For this review, take the finished solid that the model builds, in its own axes (mm). A direction names the side the tool comes from. Coordinates: 2 decimals unless noted, no trailing zeros. Loops run counter-clockwise (first coordinate to the right, second up) from the corner with the lowest first, then second, coordinate; pieces in that order, holes last. Notation, with made-up numbers: (35, 32) - (57, 32) arc R24 ccw to (57, 64) - close; hole circle Ø11 at (-9, 62). An arc over 180 degrees is marked (long way). Answer as a JSON object with one key per item and string values. Group by question number.
Item 1: We need section A-A (z = 8). Give the boundary of the cut face in (x, y).
Item 2: Tool access review of faces 1 (the cylindrical face through (41.997, -0.527, 7.395)), 2 (the flat face through (-32, -23, 10)), 3 (the flat face through (-43.77, 14.93, 7.4)): name each direction out of +Z, -Z, +X, -X, +Y, -Y from which nothing blocks a thin tool from reaching the whole face with its end or side.
Item 3: Clearance check with flat-ended pins moving along their axes: pin 1 (1.5 mm diameter, centred on y = 26.5, z = 8, fed in from +X); pin 2 (2 mm diameter, centred on y = 13, z = 7, fed in from -X); pin 3 (4 mm diameter, centred on y = 7.5, z = 6, fed in from +X). State where each tip first meets the part, or that it passes through.
Item 4: Mouldability with a two-part tool opening along X and no side actions: class faces 4 (the flat face through (-32, -23, 5)), 5 (the cylindrical face through (-36.688, -8.602, 3.623)), 6 (the cylindrical face through (-31.7, 14.62, 7.4)) as released by +X, released by -X, zero draft, split by the parting line, or undercut.
Item 5: To check wall thickness, follow line 1 (X direction, y = 7.5, z = 6.25); line 2 (X direction, y = 12.5, z = 12.5); line 3 (Y direction, x = -39, z = 1.25). State the ranges of each line that lie inside material, in increasing order.
Item 6: We need section B-B (y = 18). Give the boundary of the cut face in (x, z).
from build123d import *

# Parameters (mm, degrees)
BOSS_EXTRUDE1_DEPTH   = 15
CORTE_EXTRUS_O1_DEPTH = 5
CORTE_EXTRUS_O2_START = -10
CORTE_EXTRUS_O2_DEPTH = 5
FILETE1_R             = 10


with BuildPart() as part:
    # Sketch2 → Boss-Extrude1 (new body)
    with BuildSketch(Plane.XY):
        with BuildLine():
            Line((-40.19459236, 14.102844367), (-47.445652556, 15.776883518))
            Line((-47.445652556, 15.776883518), (-48.388260059, -2.209139093))
            Line((-48.388260059, -2.209139093), (-41.139476942, -16.435676991))
            ThreePointArc((-41.139476942, -16.435676991), (-28.61020632, -29.989765588), (-10.845255119, -35))
            Line((-10.845255119, -35), (-8, -35))
            Line((-8, -35), (19.974984355, -35))
            ThreePointArc((19.974984355, -35), (23.282173494, -34.437293044), (26.217166967, -32.8125))
            ThreePointArc((26.217166967, -32.8125), (42, 0), (26.217166967, 32.8125))
            ThreePointArc((26.217166967, 32.8125), (23.282173494, 34.437293044), (19.974984355, 35))
            Line((19.974984355, 35), (-8, 35))
            ThreePointArc((-8, 35), (-12.383711468, 33.987940463), (-15.880107536, 31.156614753))
            Line((-15.880107536, 31.156614753), (-25.000165241, 19.483473209))
            ThreePointArc((-25.000165241, 19.483473209), (-31.813223657, 14.578772972), (-40.19459236, 14.102844367))
        make_face()
    extrude(amount=BOSS_EXTRUDE1_DEPTH)

    # Esboço4 → Corte-extrusão1 (cut)
    with BuildSketch(Plane(origin=(0, 0, 0), x_dir=(-1, 0, 0), z_dir=(0, 0, -1))):
        with BuildLine():
            Line((48.388260059, -2.209139093), (27.681074333, -6.989769605))
            ThreePointArc((27.681074333, -6.989769605), (22.587110405, -9.557338795), (19.25428073, -14.186931261))
            Line((19.25428073, -14.186931261), (10.845255119, -35))
            ThreePointArc((10.845255119, -35), (28.61020632, -29.989765588), (41.139476942, -16.435676991))
            Line((41.139476942, -16.435676991), (48.388260059, -2.209139093))
        make_face()
    extrude(amount=-CORTE_EXTRUS_O1_DEPTH, mode=Mode.SUBTRACT)

    # Esboço4<2> → Corte-extrusão2 (cut)
    with BuildSketch(Plane(origin=(0, 0, 0), x_dir=(-1, 0, 0), z_dir=(0, 0, -1)).offset(CORTE_EXTRUS_O2_START)):
        with BuildLine():
            Line((48.388260059, -2.209139093), (27.681074333, -6.989769605))
            ThreePointArc((27.681074333, -6.989769605), (22.587110405, -9.557338795), (19.25428073, -14.186931261))
            Line((19.25428073, -14.186931261), (10.845255119, -35))
            ThreePointArc((10.845255119, -35), (28.61020632, -29.989765588), (41.139476942, -16.435676991))
            Line((41.139476942, -16.435676991), (48.388260059, -2.209139093))
        make_face()
    extrude(amount=-CORTE_EXTRUS_O2_DEPTH, mode=Mode.SUBTRACT)

    # Filete1
    # the kernel refuses this fillet: 10 mm, written as the material it adds along each edge
    with BuildSketch(Plane(origin=(-19.25428073, -14.186931261, 10), x_dir=(0, 0, 1), z_dir=(0.3746065934159196, -0.9271838545667843, 0))) as filete1_piece_1_section:
        with BuildLine():
            CenterArc((10, 8.660254038), FILETE1_R, 180, 60)
            Line((0, 8.660254038), (0, 0))
            Line((0, 0), (5, 0))
        make_face()
    filete1_piece_1 = extrude(amount=44.098252831, mode=Mode.PRIVATE)
    filete1_piece_1 = filete1_piece_1 & Plane(origin=(-10.845255119, -1, 11.322425454), x_dir=(-0.891006524188372, -0.4539904997395388, 0), z_dir=(0, 0, -1)) * Cylinder(34, 123, mode=Mode.PRIVATE)
    add(filete1_piece_1)
    with BuildSketch(Plane(origin=(-69.483990779, 2.661194099, 10), x_dir=(0, 0, 1), z_dir=(0.9743700647852346, -0.2249510543438682, 0))) as filete1_piece_2_section:
        with BuildLine():
            CenterArc((10, 8.660254038), FILETE1_R, 180, 60)
            Line((0, 8.660254038), (0, 0))
            Line((0, 0), (5, 0))
        make_face()
    filete1_piece_2 = extrude(amount=42.902504867, mode=Mode.PRIVATE)
    filete1_piece_2 = split(filete1_piece_2, bisect_by=Plane(origin=(-44.017931787, -10.786391272, 11.322425454), z_dir=(0.8910065241883723, 0.4539904997395381, 0)), keep=Keep.TOP, mode=Mode.PRIVATE)
    add(filete1_piece_2)
    with BuildSketch(Plane(origin=(-69.483990779, 2.661194099, 5), x_dir=(0, 0, -1), z_dir=(0.9743700647852346, -0.2249510543438682, 0))) as filete1_piece_3_section:
        with BuildLine():
            CenterArc((10, -8.660254038), FILETE1_R, 120, 60)
            Line((0, -8.660254038), (0, 0))
            Line((0, 0), (5, 0))
        make_face()
    filete1_piece_3 = extrude(amount=42.902504867, mode=Mode.PRIVATE)
    filete1_piece_3 = split(filete1_piece_3, bisect_by=Plane(origin=(-44.017931791, -10.786391265, 3.677574546), z_dir=(0.8910065241883723, 0.4539904997395381, 0)), keep=Keep.TOP, mode=Mode.PRIVATE)
    add(filete1_piece_3)
    with BuildSketch(Plane(origin=(-19.25428073, -14.186931261, 5), x_dir=(0, 0, -1), z_dir=(0.3746065934159196, -0.9271838545667843, 0))) as filete1_piece_4_section:
        with BuildLine():
            CenterArc((10, -8.660254038), FILETE1_R, 120, 60)
            Line((0, -8.660254038), (0, 0))
            Line((0, 0), (5, 0))
        make_face()
    filete1_piece_4 = extrude(amount=44.098252831, mode=Mode.PRIVATE)
    filete1_piece_4 = filete1_piece_4 & Plane(origin=(-10.845255119, -1, 3.677574546), x_dir=(-0.891006524188372, -0.4539904997395388, 0), z_dir=(0, 0, -1)) * Cylinder(34, 123, mode=Mode.PRIVATE)
    add(filete1_piece_4)
    with BuildSketch(Plane(origin=(-30.380486985, -18.682210382, 10), x_dir=(0.22495105434386828, 0.9743700647852345, 0), z_dir=(-0.9743700647852345, 0.22495105434386828, 0))) as filete1_piece_5:
        with BuildLine():
            CenterArc((3.339745962, -10), FILETE1_R, 30, 60)
            Line((3.339745962, 0), (12, 0))
            Line((12, 0), (12, -5))
        make_face()
    revolve(axis=Axis((-30.380486985, -18.682210382, 10), (0, 0, -1)), revolution_arc=55)
    with BuildSketch(Plane(origin=(-30.380486985, -18.682210382, 5), x_dir=(0.22495105434386828, 0.9743700647852345, 0), z_dir=(-0.9743700647852345, 0.22495105434386828, 0))) as filete1_piece_6:
        with BuildLine():
            CenterArc((3.339745962, 10), FILETE1_R, 270, 60)
            Line((3.339745962, 0), (12, 0))
            Line((12, 0), (12, 5))
        make_face()
    revolve(axis=Axis((-30.380486985, -18.682210382, 5), (0, 0, -1)), revolution_arc=55)


solid = part.part
Check sheet entries:
{
 "1": {"outline": "(-48.39, -2.21) - (-41.14, -16.44) arc R34 ccw to (-10.85, -35) - (19.97, -35) arc R10 ccw to (26.22, -32.81) arc R42 ccw to (26.22, 32.81) arc R10 ccw to (19.97, 35) - (-8, 35) arc R10 ccw to (-15.88, 31.16) - (-25, 19.48) arc R15 cw to (-40.19, 14.1) - (-47.45, 15.78) - close"},
 "2": {"face 1": "+Z, -Z, +X", "face 2": "+Z, -X, -Y", "face 3": "+Z, -Z, +Y"},
 "3": {"pin 1": "stops at x = 33.18", "pin 2": "stops at x = -47.64", "pin 3": "stops at x = 41.64"},
 "4": {"face 4": "zero draft", "face 5": "released by -X", "face 6": "undercut"},
 "5": {"line 1": "x = -47.88 to 41.32", "line 2": "x = -47.62 to 40.1", "line 3": "y = -5.25 to 13.88"},
 "6": {"outline": "(-26.33, 0) - (37.95, 0) - (37.95, 15) - (-26.33, 15) - close"}
}
